Solid Edge part; units mm, degrees
sketch "Sketch1" plane through (0, 0, 0) normal (1, 0, 0) x (0, 1, 0)
  line L0 (28.5, 42) -> (-28.5, 42)
  line L1 (-28.5, 42) -> (-28.5, -42)
  line L2 (-28.5, -42) -> (28.5, -42)
  line L3 (28.5, -42) -> (28.5, 42)
extrude "ExtrudedProtrusion_1" add sketch "Sketch1" against normal blind 16
sketch "Sketch2" plane through (-8, 0, -42) normal (0, 0, -1) x (-1, 0, 0)
  line L0 (-8, 28.5) -> (-33.2751, 18.6299)
  line L1 (-8, 28.5) -> (-3.9571, 28.5)
  line L2 (-3.9571, 28.5) -> (-3.9571, -28.5)
  line L3 (-3.9571, -28.5) -> (-8, -28.5)
  line L4 (-8, -28.5) -> (-33.2751, -18.6299)
  arc A0 (-33.2751, -18.6299) -> (-33.2751, 18.6299) centre (-26, 0) cw
extrude "ExtrudedProtrusion_2" add sketch "Sketch2" against normal blind 16
sketch "Sketch3" plane through (-8, 0, -42) normal (0, 0, -1) x (-1, 0, 0)
  circle A0 centre (-26, 0) radius 8
extrude "ExtrudedCutout_4" cut sketch "Sketch3" against normal blind 84.082
mirror "Mirror1" about plane through (0, 0, 0) normal (0, 0, 1) of "ExtrudedProtrusion_2"
mirror "Mirror2" about plane through (0, 0, 0) normal (0, 0, 1) of "ExtrudedCutout_4"
sketch "Sketch4" plane through (-16, 0, 0) normal (-1, 0, 0) x (0, 1, 0)
  circle A0 centre (0, 0) radius 28.3475
extrude "ExtrudedProtrusion_5" add sketch "Sketch4" along normal blind 38
extrude "Cutout1" [suppressed]
fillet "Round_3" radius 3 4 edges at (-54, -28.3475, 0) (-16, -28.3475, 0) (-16, 0, 42) (-16, 0, -42)
sketch "Sketch5" plane through (-16, 0, -26.0271) normal (-1, 0, 0) x (0, 0, 1)
  line L0 (8.0271, -4) -> (11.568, -3.9916)
  line L1 (8.0271, 4) -> (8.0271, -4)
  line L2 (11.5408, 3.8919) -> (8.0271, 4)
  arc A0 (11.5408, 3.8919) -> (11.568, -3.9916) centre (26.0271, 0) cw
extrude "ExtrudedCutout_6" cut sketch "Sketch5" along normal mid plane 204.9146
Geometry: final body of the model. Coordinates: model frame, mm. A direction names the side the tool comes from. Coordinates: 2 decimals unless noted, no trailing zeros. Order: outer loops, then holes, each group sorted by start corner. A loop starts at its lowest first (then second) coordinate and runs counter-clockwise, first axis right, second up.
1) Set-up query: faces 1 (the cylindrical face through (-33.72, -28.32, 1.25)), 2 (the cylindrical face through (38, 0, -34)), 3 (the flat face through (-16, 0, -32)). Return all of +Z, -Z, +X, -X, +Y, -Y with unobstructed straight access to the full face (end or side cutting, diameter ignored); none if empty.
Result sheet:
face 1: -X
face 2: +Z, -Z, +X
face 3: -Z, -X
2) Draft query along Y for faces 4 (the flat face through (-16, 0, 32)), 5 (the flat face through (12.8, 23.5, 34.1)), 6 (the flat face through (-27, 0, -18)), 7 (the cylindrical face through (24.349, 4.868, 34.112)). Return one class per face: released by +Y, released by -Y, zero draft, split by the parting line, or undercut.
Result sheet:
face 4: zero draft
face 5: released by +Y
face 6: undercut
face 7: undercut
3) First-contact query: P1, Ø15.5, axis at y = -2.5, z = -5, coming from the +X side; P2, Ø2.5, axis at x = -36.5, y = 0, coming from the +Z side; P3, Ø1.5, axis at y = -0.5, z = -23, coming from the +X side; P4, Ø1.5, axis at y = 0, z = -31.5, coming from the -X side. Flat tips, straight axial feed; report the tip coordinate or a pass-through.
Result sheet:
P1: passes through
P2: stops at z = 28.35
P3: stops at x = 0
P4: stops at x = -16.06
4) Section C-C (x = -34). Return loops of the section in (y, z) (1 decimal), then the cut area to 3 significant figures.
Result sheet:
outline: circle Ø56.7 at (0, 0); hole (-4, -18) - (4, -18) - (3.9, -14.5) arc R15 ccw (long way) to (-4, -14.5) - close
area: 1,790 mm2
5) Section B-B (x = 18). Return loops of the section in (y, z), then the cut area to 3 significant figures.
Result sheet:
outline: (-21.47, -42) - (-8, -42) - (-8, -26) - (-21.47, -26) - close; (-21.47, 26) - (-8, 26) - (-8, 42) - (-21.47, 42) - close; (8, -42) - (21.47, -42) - (21.47, -26) - (8, -26) - close; (8, 26) - (21.47, 26) - (21.47, 42) - (8, 42) - close
area: 862 mm2
6) Ray query, probe 1 along Z at (x, y) = (-9, 0.5); probe 2 along Z at (x, y) = (5, -16); probe 3 along X at (y, z) = (0, 37.5). Return the intervals inside material, ascending.
Result sheet:
probe 1: z = -42 to -18, 14.99 to 42
probe 2: z = -42 to -26, 26 to 42
probe 3: x = -16 to 10, 26 to 38
7) Section D-D (x = 7). Return loops of the section in (y, z), then the cut area to 3 significant figures.
Result sheet:
outline: (-25.77, -42) - (25.77, -42) - (25.77, -26) - (-25.77, -26) - close; (-25.77, 26) - (25.77, 26) - (25.77, 42) - (-25.77, 42) - close
area: 1,650 mm2
8) Section A-A (y = 0). Give the number of separate pieces and of enclosed holes in the cut face, then the cut area to 3 significant figures.
Result sheet:
separate pieces: 4
enclosed holes: 0
area: 2,420 mm2
